Model file for the job. Use its own axes, mm. Coordinates: 2 decimals unless noted, no trailing zeros. Order: outer loops, then holes, each group sorted by start corner. A loop starts at its lowest first (then second) coordinate and runs counter-clockwise, first axis right, second up. Notation, with made-up numbers: (17, 70) -> (28, 70) arc R22 ccw to (28, 108) -> close; hole circle Ø6 at (52, 52.5). An arc over 180 degrees is marked (long way). Write item = value, one per line. Start each with the question number.
Q1. Cut at D-D, the plane y = 28.5. List the corners of the cut face in (x, z), plus the area to 3 significant figures.
Q2. Cut at B-B, the plane z = 1.25. Give the number of separate pieces and of enclosed holes in the cut face, plus the area to 3 significant figures.
Q3. Flat gauge pins, fed straight in: pin 1 (2 mm diameter, centred on y = 43.5, z = 1, fed in from -X); pin 2 (1.2 mm diameter, centred on y = 41.5, z = 1, fed in from +X); pin 3 (1.2 mm diameter, centred on x = 58, z = 1, fed in from -Y). Where does each tip first touch, or does it go through?
Q4. Wall check: line 1 (X direction, y = 42, z = 3.05); line 2 (Y direction, x = -64, z = 1.3); line 3 (Y direction, x = -1.5, z = 3.7). Give the ranges that are in metal, low to high. Write a range as from..to.
Q5. Cut at A-A, the plane x = 57. List the corners of the cut face in (y, z), plus the area to 3 significant figures.
Q6. Cut at C-C, the plane x = -16.5. List the corners of the cut face in (y, z).
from build123d import *

# Parameters (mm, degrees)
BOSS_EXTRUDE2_DEPTH = 4
CUT_EXTRUDE1_DEPTH  = 4


with BuildPart() as part:
    # Sketch1 → Boss-Extrude2 (new body)
    with BuildSketch(Plane.XY):
        Polygon((-105.5, 0), (-48.5, 0), (-48.5, -7), (-26.5, -7), (-26.5, 0), (31.5, 0), (31.5, -7), (53.5, -7), (53.5, 0), (110.5, 0), (110.5, -7), (117.5, -7), (117.5, 0), (117.5, 10), (82.5, 40), (62.5, 40), (62.5, 45), (47.5, 45), (47.5, 40), (-2.5, 40), (-2.5, 45), (-22.5, 45), (-22.5, 40), (-72.5, 40), (-72.5, 45), (-92.5, 45), (-92.5, 40), (-117.5, 40), (-117.5, 0), (-117.5, -7), (-105.5, -7), align=None)
    extrude(amount=BOSS_EXTRUDE2_DEPTH)

    # Sketch2 → Cut-Extrude1 (cut)
    with BuildSketch(Plane.XY.offset(4)):
        Polygon((-71.5, 20), (-71.5, 24.3), (-57.5, 24.3), (-57.5, 15.7), (-71.5, 15.7), align=None)
        Polygon((52.5, 20), (52.5, 24.3), (66.5, 24.3), (66.5, 15.7), (52.5, 15.7), align=None)
    extrude(amount=-CUT_EXTRUDE1_DEPTH, mode=Mode.SUBTRACT)


solid = part.part
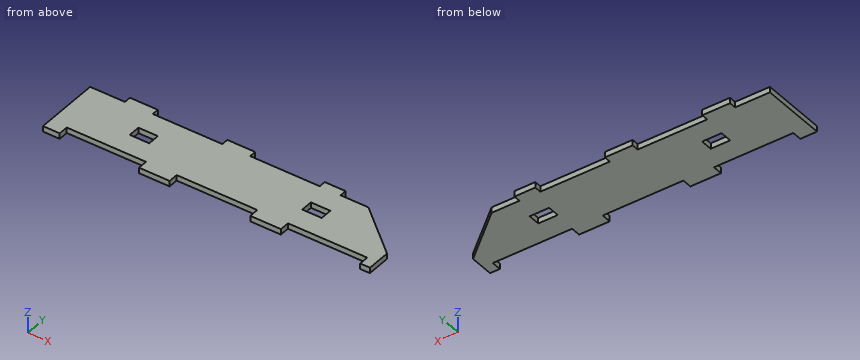
Here are the results:
q1.outline = (-117.5, 0) -> (95.92, 0) -> (95.92, 4) -> (-117.5, 4) -> close
q1.area = 854 mm²
q2.separate_pieces = 1
q2.enclosed_holes = 2
q2.area = 9,350 mm²
q3.pin_1 = -92.5
q3.pin_2 = 62.5
q3.pin_3 = 0
q4.line_1 = -92.5..-72.5, -22.5..-2.5, 47.5..62.5
q4.line_2 = 0..15.7, 24.3..40
q4.line_3 = 0..40
q5.outline = (0, 0) -> (15.7, 0) -> (15.7, 4) -> (0, 4) -> close; (24.3, 0) -> (45, 0) -> (45, 4) -> (24.3, 4) -> close
q5.area = 146 mm²
q6.outline = (0, 0) -> (45, 0) -> (45, 4) -> (0, 4) -> close
